Part model, mm, in its own coordinate system. Face numbers are marked on the shaded views. A direction names the side the tool comes from. Round coordinates to 2 decimals unless told otherwise and drop trailing zeros. Loops run counter-clockwise (first coordinate to the right, second up) from the corner with the lowest first, then second, coordinate; pieces in that order, holes last. Notation, with made-up numbers: M -28.75,-25.5 L -9.75,-25.5 A20 ccw -9.75,11.5 Z; hole C 65,-36 d9. An arc over 180 degrees is marked long. Answer as CSV lines item,"result". Start each with the question number.
Item 1: Band-saw the part on D-D (y = -58.5). Give the cut face in (x, z), and give its area (3 significant figures).
Item 2: Which spindle directions (+Z, -Z, +X, -X, +Y, -Y) get a long thin tool onto all of the face, cutting with end or side? Do the marked faces 1 and 2. Say none if no direction does.
Item 3: Wall check: line 1 (Z direction, x = -0.25, y = -34.5); line 2 (X direction, y = -24.5, z = -2); line 3 (Z direction, x = -0.15, y = -4). Give the ranges that are in metal, low to high.
Item 4: Band-saw the part on C-C (x = 0.75). Give the cut face in (y, z).
Item 5: Band-saw the part on A-A (y = -4). Give the cut face in (x, z).
Item 6: Mould opens along Y. For the marked faces 3, 4 and 5 say: pulls with the +Y half, pulls with the -Y half, needs draft (parallel to the pull), parting line crosses it, or undercut.
Item 7: Band-saw the part on B-B (z = -0.75). Give the cut face in (x, y).
Item 8: Drop flat-ended pins along their axis: pin 1 Ø2.5 at (x, z) = (3.5, -1) entering from +Y; pin 2 Ø2.5 at (y, z) = (-8, 1.5) entering from +X; pin 3 Ø1 at (x, y) = (1, -56.5) entering from +Z. Give the stop position or say it passes through.
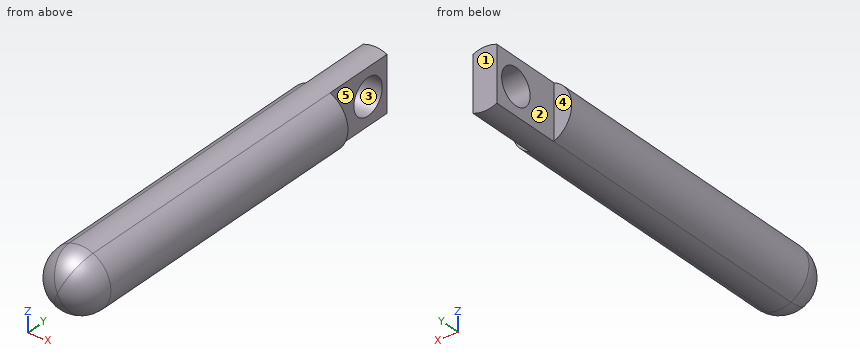
```python
from build123d import *

# Parameters (mm, degrees)
F2_DEPTH = 67
F3_DEPTH = 12
F4_R     = 3
F5_DEPTH = 25
F6_R     = 5


with BuildPart() as f2:
    # F1 (on Front) → F2 (new body)
    with BuildSketch(Plane.XZ):
        with BuildLine():
            ThreePointArc((2, -4.582575695), (4.1833001327, -2.7386127875), (5, 0))
            ThreePointArc((5, 0), (4.1833001327, 2.7386127875), (2, 4.582575695))
            Line((2, 4.582575695), (2, -4.582575695))
        make_face()
        with BuildLine():
            Line((2, -4.582575695), (2, 4.582575695))
            ThreePointArc((2, 4.582575695), (0, 5), (-2, 4.582575695))
            Line((-2, 4.582575695), (-2, -4.582575695))
            ThreePointArc((-2, -4.582575695), (0, -5), (2, -4.582575695))
        make_face()
        with BuildLine():
            Line((-2, -4.582575695), (-2, 4.582575695))
            ThreePointArc((-2, 4.582575695), (-5, 0), (-2, -4.582575695))
        make_face()
    extrude(amount=F2_DEPTH)

    # F1 (on Front) → F3 (cut)
    with BuildSketch(Plane.XZ):
        with BuildLine():
            Line((-2, -4.582575695), (-2, 4.582575695))
            ThreePointArc((-2, 4.582575695), (-5, 0), (-2, -4.582575695))
        make_face()
        with BuildLine():
            ThreePointArc((2, -4.582575695), (4.1833001327, -2.7386127875), (5, 0))
            ThreePointArc((5, 0), (4.1833001327, 2.7386127875), (2, 4.582575695))
            Line((2, 4.582575695), (2, -4.582575695))
        make_face()
    extrude(amount=F3_DEPTH, mode=Mode.SUBTRACT)

    # F4 (on face) → F5 (cut)
    with BuildSketch(Plane.YZ.offset(2)):
        with Locations((-4, 0)):
            Circle(F4_R)
    extrude(amount=-F5_DEPTH, mode=Mode.SUBTRACT)

    # F6
    f6_edges = [f2.edges().sort_by_distance(p)[0] for p in [
        (2, -67, -4.582576),
    ]]
    fillet(f6_edges, radius=F6_R)


solid = f2.part
```
Answer block:
1,outline,"C 0,0 d10"
1,area,"78.5 mm^2"
2,face 1,"+Z, -Z, +X, -X, +Y"
2,face 2,"+Z, -Z, -X, +Y"
3,line 1,"z = -4.99 to 4.99"
3,line 2,"x = -4.58 to 4.58"
3,line 3,"z = -5 to -3, 3 to 5"
4,outline,"M -62,-4.94 L 0,-4.94 L 0,4.94 L -62,4.94 A4.94 ccw Z; hole C -4,0 d6"
5,outline,"M -2,-4.58 A5 ccw 2,-4.58 L 2,-3 L -2,-3 Z; M -2,3 L 2,3 L 2,4.58 A5 ccw -2,4.58 Z"
6,face 3,"undercut"
6,face 4,"pulls with the +Y half"
6,face 5,"needs draft"
7,outline,"M -4.94,-62 A4.94 ccw 4.94,-62 L 4.94,-12 L 2,-12 L 2,-6.9 L -2,-6.9 L -2,-12 L -4.94,-12 Z; M -2,-1.1 L 2,-1.1 L 2,0 L -2,0 Z"
8,pin 1,"stops at y = -12"
8,pin 2,"stops at x = 2"
8,pin 3,"stops at z = 4.97"
